Geometry check sheet. Reference: the model listing, model coordinates, mm. A direction names the side the tool comes from. Give positions to 0.01 mm unless a question says otherwise; leave off trailing zeros. Order: outer loops, then holes, each group sorted by start corner. A loop starts at its lowest first (then second) coordinate and runs counter-clockwise, first axis right, second up. Notation, with made-up numbers: M -36,-31 L 1,-31 A10 ccw 1,-15 Z; hole C -5,60 d1. An arc over 180 degrees is marked long. Answer as CSV lines item,"result".
from build123d import *

# Parameters (mm, degrees)
SKETCH1_R           = 10
BOSS_EXTRUDE1_DEPTH = 10
BOSS_EXTRUDE2_DEPTH = 5


with BuildPart() as part:
    # Sketch1 → Boss-Extrude1 (new, symmetric)
    with BuildSketch(Plane.XY):
        with BuildLine():
            ThreePointArc((-22, 75.198039027), (0, 65.594117082), (22, 75.198039027))
            ThreePointArc((22, 75.198039027), (46.234544698, 72.060228511), (35.344077706, 50.184288755))
            ThreePointArc((35.344077706, 50.184288755), (13.282230039, 34.133637057), (13.344077706, 6.850955421))
            ThreePointArc((13.344077706, 6.850955421), (0, -15), (-13.344077706, 6.850955421))
            ThreePointArc((-13.344077706, 6.850955421), (-13.282230039, 34.133637057), (-35.344077706, 50.184288755))
            ThreePointArc((-35.344077706, 50.184288755), (-46.234544698, 72.060228511), (-22, 75.198039027))
        make_face()
        Circle(SKETCH1_R, mode=Mode.SUBTRACT)
        with Locations((-33, 65)):
            Circle(SKETCH1_R, mode=Mode.SUBTRACT)
        with Locations((33, 65)):
            Circle(SKETCH1_R, mode=Mode.SUBTRACT)
    extrude(amount=BOSS_EXTRUDE1_DEPTH, both=True)

    # Sketch1_3 → Boss-Extrude2 (add, symmetric)
    with BuildSketch(Plane.XY):
        with BuildLine():
            ThreePointArc((33, 85), (50.045189115, 75.462386346), (50.833335385, 55.946152804))
            Line((50.833335385, 55.946152804), (17.833335385, -9.053847196))
            ThreePointArc((17.833335385, -9.053847196), (0, -20), (-17.833335385, -9.053847196))
            Line((-17.833335385, -9.053847196), (-50.833335385, 55.946152804))
            ThreePointArc((-50.833335385, 55.946152804), (-50.045189115, 75.462386346), (-33, 85))
            Line((-33, 85), (33, 85))
        make_face()
        with BuildLine():
            ThreePointArc((-22, 75.198039027), (-46.234544698, 72.060228511), (-35.344077706, 50.184288755))
            ThreePointArc((-35.344077706, 50.184288755), (-13.282230039, 34.133637057), (-13.344077706, 6.850955421))
            ThreePointArc((-13.344077706, 6.850955421), (0, -15), (13.344077706, 6.850955421))
            ThreePointArc((13.344077706, 6.850955421), (13.282230039, 34.133637057), (35.344077706, 50.184288755))
            ThreePointArc((35.344077706, 50.184288755), (46.234544698, 72.060228511), (22, 75.198039027))
            ThreePointArc((22, 75.198039027), (0, 65.594117082), (-22, 75.198039027))
        make_face(mode=Mode.SUBTRACT)
    extrude(amount=BOSS_EXTRUDE2_DEPTH, both=True)


solid = part.part
(1) Section check B-B on z = 1.5. Enter the section's corners in (x, y).
The answers:
outline,"M -50.83,55.95 L -17.83,-9.05 A20 ccw 17.83,-9.05 L 50.83,55.95 A20 ccw 33,85 L -33,85 A20 ccw Z; hole C -33,65 d20; hole C 0,0 d20; hole C 33,65 d20"
(2) Draft check along Y on faces 6 (the face through (13.464, 34.486, 7.535)), 7 (the face through (-0.346, 65.596, -7.465)), 8 (the face through (46.04, 72.41, 7.54)). Enter one of: +Y half, -Y half, draft (parallel to the pull), parting line (faces both ways), or undercut.
The answers:
face 6,"undercut"
face 7,"+Y half"
face 8,"parting line"
(3) Section check A-A on x = 0. Enter the section's corners in (y, z).
The answers:
outline,"M -20,-5 L -15,-5 L -15,-10 L -10,-10 L -10,10 L -15,10 L -15,5 L -20,5 Z; M 10,-10 L 65.59,-10 L 65.59,-5 L 85,-5 L 85,5 L 65.59,5 L 65.59,10 L 10,10 Z"
(4) Section check D-D on y = 15.5. Enter the section's corners in (x, z).
The answers:
outline,"M -30.3,-5 L -10.46,-5 L -10.46,-10 L 10.46,-10 L 10.46,-5 L 30.3,-5 L 30.3,5 L 10.46,5 L 10.46,10 L -10.46,10 L -10.46,5 L -30.3,5 Z"
(5) Gauge pin test, flat ends, axial feed: P1, Ø1, axis at x = 33.5, z = -3, coming from the -Y side; P2, Ø4, axis at y = 22, z = 2.5, coming from the -X side; P3, Ø4, axis at x = -21, y = 11.5, coming from the -Z side. Record the tip position at first contact, or that the pin passes through.
The answers:
P1,"stops at y = 20.82"
P2,"stops at x = -34.61"
P3,"stops at z = -5"
(6) Material ranges on line 1 (X direction, y = 73.5, z = 1.75); line 2 (Z direction, x = -25, y = 78); line 3 (Y direction, x = 0.5, z = -7), recorded low to high.
The answers:
line 1,"x = -51.1 to -38.27, -27.73 to 27.73, 38.27 to 51.1"
line 2,"z = -5 to 5"
line 3,"y = -14.99 to -9.99, 9.99 to 65.6"
(7) Tool access check on faces 1 (the face through (13.464, 34.486, -7.465)), 2 (the face through (-13.105, 33.779, 7.535)), 3 (the face through (-12, 29, 5)), 4 (the face through (-13.105, 33.779, -7.465)), 5 (the face through (-46.42, 71.7, -7.46)). Record the directions out of +Z, -Z, +X, -X, +Y, -Y that give a thin tool (end or side, any length) a straight path to the whole face; none if there is none.
The answers:
face 1,"-Z, +X"
face 2,"+Z, -X"
face 3,"+Z"
face 4,"-Z, -X"
face 5,"-Z"
(8) Section check C-C on y = 0. Enter the section's corners in (x, z).
The answers:
outline,"M -22.43,-5 L -15,-5 L -15,-10 L -10,-10 L -10,10 L -15,10 L -15,5 L -22.43,5 Z; M 10,-10 L 15,-10 L 15,-5 L 22.43,-5 L 22.43,5 L 15,5 L 15,10 L 10,10 Z"
